Geometry check sheet. Reference: the model listing, model coordinates, mm. A direction names the side the tool comes from. Round coordinates to 2 decimals unless told otherwise and drop trailing zeros. Loops run counter-clockwise (first coordinate to the right, second up) from the corner with the lowest first, then second, coordinate; pieces in that order, holes last.
```python
from build123d import *

# Parameters (mm, degrees)
SKETCH1_R           = 2.1
BOSS_EXTRUDE1_DEPTH = 5


with BuildPart() as part:
    # Sketch1 → Boss-Extrude1 (new body)
    with BuildSketch(Plane.XY):
        with BuildLine():
            Line((156.630765815, 0), (0, 0))
            Line((0, 0), (17.930632383, -38.452365235))
            ThreePointArc((17.930632383, -38.452365235), (25.310795957, -46.867828916), (36.056788124, -50))
            Line((36.056788124, -50), (120.573977692, -50))
            ThreePointArc((120.573977692, -50), (131.319969859, -46.867828916), (138.700133432, -38.452365235))
            Line((138.700133432, -38.452365235), (156.630765815, 0))
        make_face()
        with Locations((148.315382907, -5)):
            Circle(SKETCH1_R, mode=Mode.SUBTRACT)
        with Locations((8.315382909, -5)):
            Circle(SKETCH1_R, mode=Mode.SUBTRACT)
        with BuildLine():
            Line((118.315382908, -15), (38.315382908, -15))
            ThreePointArc((38.315382908, -15), (25.815382908, -27.5), (38.315382908, -40))
            Line((38.315382908, -40), (118.315382908, -40))
            ThreePointArc((118.315382908, -40), (130.815382908, -27.5), (118.315382908, -15))
        make_face(mode=Mode.SUBTRACT)
    extrude(amount=BOSS_EXTRUDE1_DEPTH)


solid = part.part
```
1) Scan lines: line 1 along Y through (x, z) = (41, 1.8); line 2 along X through (y, z) = (-23, 3.75); line 3 along X through (y, z) = (-16, 2.75). Record each from-to range of solid material in increasing order.
Report:
line 1: y = -50 to -40, -15 to 0
line 2: x = 10.73 to 26.65, 129.98 to 145.91
line 3: x = 7.46 to 33.42, 123.21 to 149.17
2) Sectioned sample at C-C, the plane x = 96. Record the cut outline in (y, z), then the cut area to 3 significant figures.
Report:
outline: (-50, 0) - (-40, 0) - (-40, 5) - (-50, 5) - close; (-15, 0) - (0, 0) - (0, 5) - (-15, 5) - close
area: 125 mm2
3) Mould release check, pull along X, two halves, no side actions. Record for faces 3 (the face through (147.54, -19.495, 2.465)), 4 (the face through (25.82, -27.23, 2.46)), 5 (the face through (78, -50, 2)): +X half, -X half, draft (parallel to the pull), parting line (faces both ways), or undercut.
Report:
face 3: +X half
face 4: undercut
face 5: draft
4) Sectioned sample at A-A, the plane y = -5. Record the cut outline in (x, z), then the cut area to 3 significant figures.
Report:
outline: (2.33, 0) - (6.22, 0) - (6.22, 5) - (2.33, 5) - close; (10.42, 0) - (146.22, 0) - (146.22, 5) - (10.42, 5) - close; (150.42, 0) - (154.3, 0) - (154.3, 5) - (150.42, 5) - close
area: 718 mm2
5) Sectioned sample at D-D, the plane y = -26.5. Record the cut outline in (x, z), then the cut area to 3 significant figures.
Report:
outline: (12.36, 0) - (25.86, 0) - (25.86, 5) - (12.36, 5) - close; (130.78, 0) - (144.27, 0) - (144.27, 5) - (130.78, 5) - close
area: 135 mm2
6) Sectioned sample at B-B, the plane z = 2.9. Record the cut outline in (x, y).
Report:
outline: (0, 0) - (17.93, -38.45) arc R20 ccw to (36.06, -50) - (120.57, -50) arc R20 ccw to (138.7, -38.45) - (156.63, 0) - close; hole circle Ø4.2 at (8.32, -5); hole (38.32, -40) - (118.32, -40) arc R12.5 ccw to (118.32, -15) - (38.32, -15) arc R12.5 ccw to start; hole circle Ø4.2 at (148.32, -5)
7) Access from +Z, -Z, +X, -X, +Y, -Y to the whole of each face (thin tool, end or side, straight path). Record for faces 1 (the face through (79, -15, 2)), 2 (the face through (25.177, -46.782, 2.465)).
Report:
face 1: +Z, -Z
face 2: +Z, -Z, -X, -Y
